Build history of the part. All positions in model axes, mm. Give positions to 0.01 mm unless a question says otherwise; leave off trailing zeros. Order: outer loops, then holes, each group sorted by start corner. A loop starts at its lowest first (then second) coordinate and runs counter-clockwise, first axis right, second up. Notation, with made-up numbers: (-22, 30.25) - (21, 30.25) arc R21 ccw to (21, 66.25) - close; hole circle Ø1 at (3.25, 11.25). An arc over 180 degrees is marked (long way). Use a Markdown table: item, result. Add a question column.
(1) Flat gauge pins, fed straight in: pin 1 (2 mm diameter, centred on x = 5, z = 0, fed in from +Y); pin 2 (1.5 mm diameter, centred on x = 3, y = -8, fed in from +Z). Where does each tip first touch, or does it go through?
(2) Slice it at B-B (y = 9.5). Write the cut outline in (x, z), then the cut area to 3 significant figures.
(3) Wall check: line 1 (Z direction, x = 5, y = 12.75); line 2 (X direction, y = 9, z = -42); line 3 (Y direction, x = 3, z = 30) (3 decimals). Give the ranges that are in metal, low to high.
(4) Slice it at C-C (x = 1.5). Write the cut outline in (y, z) (3 decimals).
(5) Slice it at A-A (y = 5). Write the cut outline in (x, z) (3 decimals), then the cut area to 3 significant figures.
(6) Slice it at D-D (y = -10). Write the cut outline in (x, z), then the cut area to 3 significant figures.
from build123d import *

# Parameters (mm, degrees)
SKETCH1_W                     = 100
SKETCH1_H                     = 30
SKETCH1_R                     = 3.175
BOSS_EXTRUDE1_DEPTH           = 10
FILLET1_R                     = 15
CBORE_FOR_M3_SHCS_D           = 3.4
CBORE_FOR_M3_SHCS_DEPTH       = 23
CBORE_FOR_M3_SHCS_CBORE_D     = 6.5
CBORE_FOR_M3_SHCS_CBORE_DEPTH = 3
CBORE_FOR_M3_SHCS_TIP         = 1.021463052


with BuildPart() as part:
    # Sketch1 → Boss-Extrude1 (new body)
    with BuildSketch(Plane(origin=(0, 0, 0), x_dir=(0, 0, -1), z_dir=(1, 0, 0))):
        Rectangle(SKETCH1_W, SKETCH1_H)
        with Locations((-30, 5)):
            Circle(SKETCH1_R, mode=Mode.SUBTRACT)
    extrude(amount=BOSS_EXTRUDE1_DEPTH)

    # Fillet1
    fillet1_edges = [part.edges().sort_by_distance(p)[0] for p in [
        (5, -15, 50),
    ]]
    fillet(fillet1_edges, radius=FILLET1_R)

    # CBORE for M3 SHCS
    with Locations(Plane(origin=(-616.293536786, 25, -1323.282701689), x_dir=(1, 0, 0), z_dir=(0, 1, 0))):
        with Locations((731.293536786, -1281.282701689), (731.293536786, -1359.282701689), (621.293536786, -1281.282701689), (621.293536786, -1365.282701689), (621.293536786, -1323.282701689), (731.293536786, -1320.282701689)):
            CounterBoreHole(CBORE_FOR_M3_SHCS_D / 2, CBORE_FOR_M3_SHCS_CBORE_D / 2, CBORE_FOR_M3_SHCS_CBORE_DEPTH, depth=CBORE_FOR_M3_SHCS_DEPTH)
            with Locations((0, 0, -(CBORE_FOR_M3_SHCS_DEPTH + CBORE_FOR_M3_SHCS_TIP / 2))):  # 118° drill point
                Cone(0, CBORE_FOR_M3_SHCS_D / 2, CBORE_FOR_M3_SHCS_TIP, mode=Mode.SUBTRACT)


solid = part.part
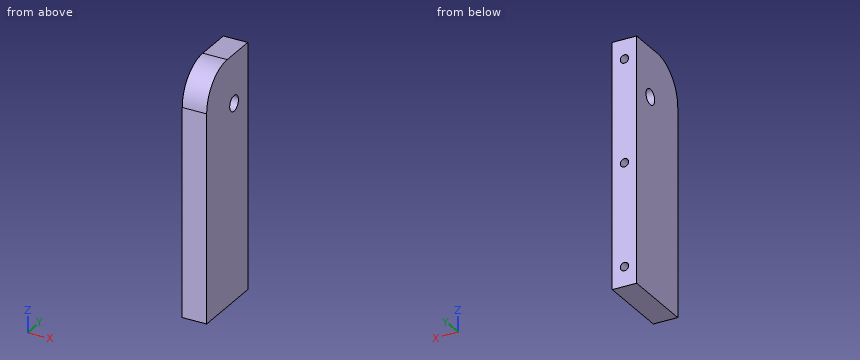
Solution:
| question | item | result |
|---|---|---|
| 1 | pin 1 | y = 1.58 |
| 1 | pin 2 | z = 48.13 |
| 2 | outline | (0, -50) - (10, -50) - (10, 50) - (0, 50) - close; hole circle Ø3.4 at (5, -42); hole circle Ø3.4 at (5, 0); hole circle Ø3.4 at (5, 42) |
| 2 | area | 973 mm2 |
| 3 | line 1 | -50 to -43.7, -40.3 to -1.7, 1.7 to 40.3, 43.7 to 50 |
| 3 | line 2 | 0 to 3.3, 6.7 to 10 |
| 3 | line 3 | -15 to 1.825, 8.175 to 15 |
| 4 | outline | (-15, -50) - (15, -50) - (15, 50) - (0, 50) arc R15 ccw to (-15, 35) - close; hole circle Ø6.35 at (5, 30) |
| 5 | outline | (0, -50) - (10, -50) - (10, 26.825) - (0, 26.825) - close; (0, 33.175) - (10, 33.175) - (10, 50) - (0, 50) - close; hole circle Ø3.4 at (5, -42); hole circle Ø3.4 at (5, 0); hole circle Ø3.4 at (5, 42) |
| 5 | area | 909 mm2 |
| 6 | outline | (0, -50) - (10, -50) - (10, 46.18) - (0, 46.18) - close |
| 6 | area | 962 mm2 |
